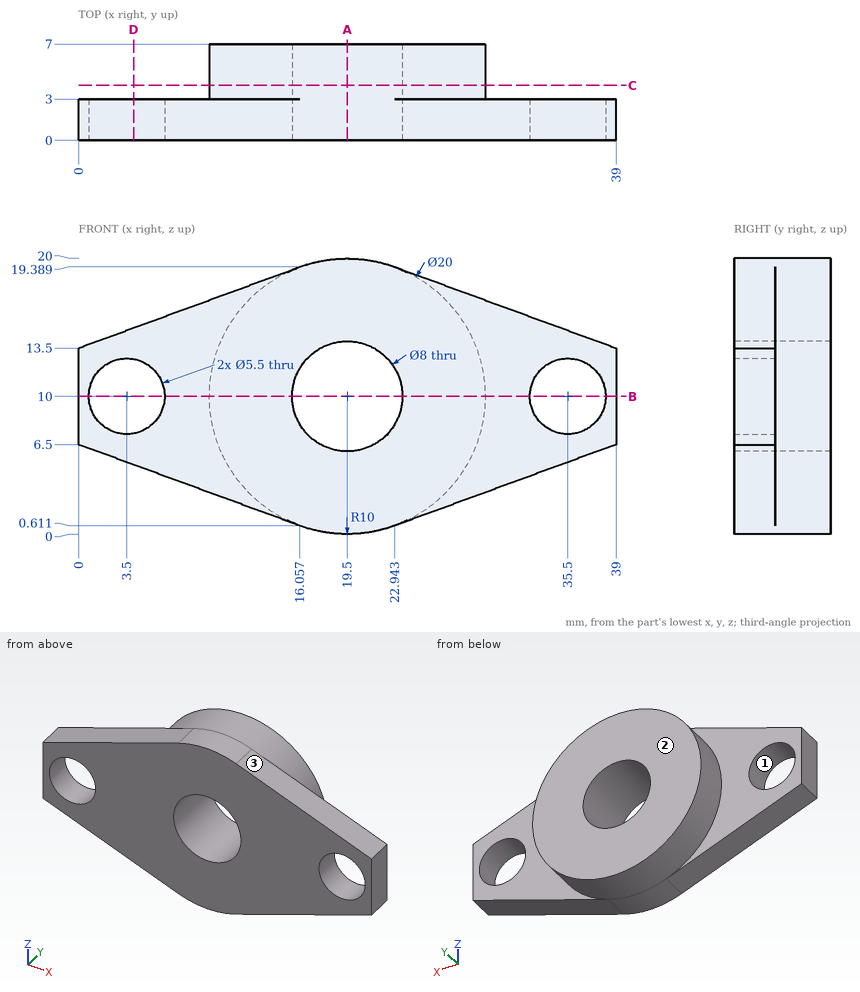
Geometry check sheet. Reference: drawing and pictorial views, mm from the part's lowest x, y, z. Give positions to 0.01 mm unless a question says otherwise; leave off trailing zeros. Loops run counter-clockwise (first coordinate to the right, second up) from the corner with the lowest first, then second, coordinate; pieces in that order, holes last. Notation, with made-up numbers: (53.25, 5.25) - (64.25, 5.25) arc R30 cw to (64.25, 43.25) - close; hole circle Ø2 at (5.5, 44). An arc over 180 degrees is marked (long way). One line per question, with ' | ' between items. Start each with the question number.
1. Cross-section at D-D, the plane x = 4. Enter the section's corners in (y, z) (1 decimal), plus the area to 3 significant figures.
2. Cross-section at C-C, the plane y = 4. Enter the section's corners in (x, z).
3. Cross-section at B-B, the plane z = 10. Enter the section's corners in (x, y), plus the area to 3 significant figures.
4. Draft check along X on the marked faces 1, 2 and 3. Enter one of: released by +X, released by -X, zero draft, split by the parting line, or undercut.
5. Cross-section at A-A, the plane x = 19.5. Enter the section's corners in (y, z).
6. Gauge pin test, flat ends, axial feed: pin 1 Ø4.5 at (x, z) = (3.5, 10) entering from -Y; pin 2 Ø1.5 at (y, z) = (6, 5) entering from +X; pin 3 Ø5 at (x, z) = (6.5, 12) entering from +Y. Record the tip position at first contact, or that the pin passes through.
7. Material ranges on line 1 along X through (y, z) = (1.15, 10); line 2 along Y through (x, z) = (2, 7); line 3 along X through (y, z) = (4, 10), recorded low to high. Write a range as [from, to].
Check result:
1) outline: (0, 5) - (3, 5) - (3, 7.3) - (0, 7.3) - close; (0, 12.7) - (3, 12.7) - (3, 15) - (0, 15) - close | area: 13.6 mm2
2) outline: circle Ø20 at (19.5, 10); hole circle Ø8 at (19.5, 10)
3) outline: (0, 0) - (0.75, 0) - (0.75, 3) - (0, 3) - close; (6.25, 0) - (15.5, 0) - (15.5, 7) - (9.5, 7) - (9.5, 3) - (6.25, 3) - close; (23.5, 0) - (32.75, 0) - (32.75, 3) - (29.5, 3) - (29.5, 7) - (23.5, 7) - close; (38.25, 0) - (39, 0) - (39, 3) - (38.25, 3) - close | area: 108 mm2
4) face 1: undercut | face 2: zero draft | face 3: released by +X
5) outline: (0, 0) - (7, 0) - (7, 6) - (0, 6) - close; (0, 14) - (7, 14) - (7, 20) - (0, 20) - close
6) pin 1: passes through | pin 2: stops at x = 28.55 | pin 3: stops at y = 3
7) line 1: x = [0, 0.75], [6.25, 15.5], [23.5, 32.75], [38.25, 39] | line 2: y = [0, 3] | line 3: x = [9.5, 15.5], [23.5, 29.5]
